The model under review builds one solid part; all positions refer to its coordinate system, in mm. A direction names the side the tool comes from. Coordinates: 2 decimals unless noted, no trailing zeros. Order: outer loops, then holes, each group sorted by start corner. A loop starts at its lowest first (then second) coordinate and runs counter-clockwise, first axis right, second up. Notation, with made-up numbers: (41, -18.75) -> (95, -18.75) arc R21 cw to (95, -12.75) -> close; hole circle Ø6 at (-33, 11). An arc over 180 degrees is marked (long way). Use one line per item in the form item = value. Start each with the question number.
(1) Mouldability with a two-part tool opening along Z and no side actions: class faces 4 (the cylindrical face through (7.518, 242.871, 4.93)), 5 (the flat face through (187, 127, 10)), 6 (the flat face through (187, 127, 0)) as +Z half, -Z half, draft (parallel to the pull), parting line (faces both ways), or undercut.
(2) Insertion check: pin 1 Ø5 at (y, z) = (-7.5, 7) entering from -X; pin 2 Ø3 at (x, z) = (316, 3.5) entering from -Y; pin 3 Ø4 at (y, z) = (17.5, 3.5) entering from +X. Each pin has a flat end and moves straight along its axis. Give the tip position at first contact, or say it passes through.
(3) Take a section at C-C (x = 174). State the section outline as (y, z) points, then the cut area to 3 significant figures.
(4) Take a section at B-B (y = 254). State the section outline as (x, z) points, then the cut area to 3 significant figures.
(5) Wall thickness on line 1 along Y through (x, z) = (265, 6.75); line 2 along Y through (x, z) = (238, 4); line 3 along X through (y, z) = (-15.5, 5): over which ranges is each line inside the solid? List them lowest first.
(6) Take a section at A-A (z = 7.75). State how many separate pieces and enclosed holes the cut face has, then the cut area to 3 significant figures.
(7) For faces 1 (the flat face through (220, -10, 5)), 2 (the flat face through (59, 250, 5)), 3 (the flat face through (302, 0, 5)), list the 3-axis set-ups (+Z, -Z, +X, -X, +Y, -Y) from which the entire face can be reached by the end or side of a thin tool; tool diameter is ignored.
```python
from build123d import *

# Parameters (mm, degrees)
F1_DEPTH = 10
F2_R     = 3.5
F3_DEPTH = 25
F4_R     = 3.1
F5_DEPTH = 25


with BuildPart() as f1:
    # F0 (on Top) → F1 (new body)
    with BuildSketch(Plane.XY):
        with BuildLine():
            ThreePointArc((0, 25), (7.32233, 7.32233), (25, 0))
            Line((25, 0), (91.562498, 0))
            Line((91.562498, 0), (95, 5))
            Line((95, 5), (98.437502, 0))
            Line((98.437502, 0), (220, 0))
            Line((220, 0), (220, -20))
            ThreePointArc((220, -20), (224.393398, -30.606602), (235, -35))
            ThreePointArc((235, -35), (245.606602, -30.606602), (250, -20))
            Line((250, -20), (250, 0))
            Line((250, 0), (355, 0))
            ThreePointArc((355, 0), (372.67767, 7.32233), (380, 25))
            Line((380, 25), (380, 225))
            ThreePointArc((380, 225), (372.67767, 242.67767), (355, 250))
            Line((355, 250), (250, 250))
            Line((250, 250), (250, 270))
            ThreePointArc((250, 270), (245.606602, 280.606602), (235, 285))
            ThreePointArc((235, 285), (224.393398, 280.606602), (220, 270))
            Line((220, 270), (220, 250))
            Line((220, 250), (98.437502, 250))
            Line((98.437502, 250), (95, 245))
            Line((95, 245), (91.562498, 250))
            Line((91.562498, 250), (25, 250))
            ThreePointArc((25, 250), (7.32233, 242.67767), (0, 225))
            Line((0, 225), (0, 25))
        make_face()
    extrude(amount=F1_DEPTH)

    # F2 (on face) → F3 (cut)
    with BuildSketch(Plane.XY.offset(10)):
        with Locations((235, -20)):
            Circle(F2_R)
        with Locations((235, 270)):
            Circle(F2_R)
    extrude(amount=-F3_DEPTH, mode=Mode.SUBTRACT)

    # F4 (on face) → F5 (cut)
    with BuildSketch(Plane.XY.offset(10)):
        with Locations((265, 215)):
            Circle(F4_R)
        with Locations((265, 125)):
            Circle(F4_R)
        with Locations((265, 35)):
            Circle(F4_R)
        with Locations((365, 45)):
            Circle(F4_R)
        with Locations((365, 125)):
            Circle(F4_R)
        with Locations((365, 205)):
            Circle(F4_R)
    extrude(amount=-F5_DEPTH, mode=Mode.SUBTRACT)


solid = f1.part
```
Findings:
q1.face_4 = draft
q1.face_5 = +Z half
q1.face_6 = -Z half
q2.pin_1 = 220
q2.pin_2 = 0
q2.pin_3 = 379.39
q3.outline = (0, 0) -> (250, 0) -> (250, 10) -> (0, 10) -> close
q3.area = 2,500 mm²
q4.outline = (220, 0) -> (250, 0) -> (250, 10) -> (220, 10) -> close
q4.area = 300 mm²
q5.line_1 = 0 to 31.9, 38.1 to 121.9, 128.1 to 211.9, 218.1 to 250
q5.line_2 = -34.7 to -21.8, -18.2 to 268.2, 271.8 to 284.7
q5.line_3 = 220 to 250
q6.separate_pieces = 1
q6.enclosed_holes = 8
q6.area = 96,100 mm²
q7.face_1 = +Z, -Z, -X, -Y
q7.face_2 = +Z, -Z, -X, +Y
q7.face_3 = +Z, -Z, +X, -Y
